The model under review builds one solid part; all positions refer to its coordinate system, in mm. Face numbers are marked on the shaded views. A direction names the side the tool comes from. Coordinates: 2 decimals unless noted, no trailing zeros. Loops run counter-clockwise (first coordinate to the right, second up) from the corner with the lowest first, then second, coordinate; pieces in that order, holes last. Notation, with made-up numbers: M 12.5,54.5 L 42.5,54.5 A37 cw 42.5,93.5 Z; hole C -36,85.5 d7. An arc over 180 degrees is marked long. Return JSON: item names as keys, results as strings.
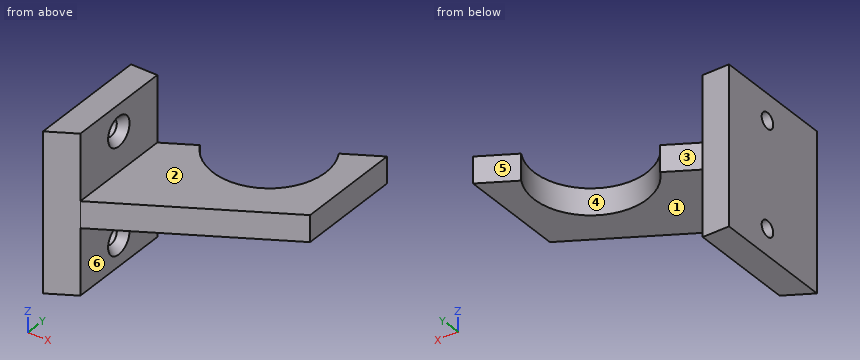
Autodesk Inventor part; units mm, degrees
ref_plane "YZ Plane" through (0, 0, 0) normal (1, 0, 0) x (0, 1, 0)
ref_plane "XZ Plane" through (0, 0, 0) normal (0, 1, 0) x (-1, 0, 0)
ref_plane "XY Plane" through (0, 0, 0) normal (0, 0, 1) x (1, 0, 0)
sketch "Sketch5" plane through (0, 0, 0) normal (0, 0, 1) x (1, 0, 0)
  line L0 (0, 0) -> (6.35, 0)
  line L1 (6.35, 0) -> (6.35, 25.4)
  line L2 (6.35, 25.4) -> (0, 25.4)
  line L3 (0, 25.4) -> (0, 0)
  dimension "d21" = 25.4
  dimension "d22" = 6.35
extrude "Extrusion3" add sketch "Sketch5" against normal mid plane 38.1
sketch "Sketch6" plane through (0, 0, 0) normal (0, 0, 1) x (1, 0, 0)
  line L0 (6.35, 25.4) -> (6.35, 0)
  line L1 (0, 25.4) -> (6.35, 25.4)
  line L2 (6.35, 0) -> (0, 0)
  line L3 (0, 0) -> (0, 25.4)
  line L4 (6.35, 0) -> (45.4025, 22.547)
  line L5 (6.35, 0) -> (51.4439, 0) construction
  line L6 (45.4025, 47.947) -> (45.4025, 22.547)
  arc A0 (13.5766, 29.5723) -> (37.2234, 43.2248) centre (25.4, 36.3985) ccw
  line L7 (6.35, 25.4) -> (13.5766, 29.5723)
  line L8 (37.2234, 43.2248) -> (45.4025, 47.947)
  dimension "d25" = 30
  dimension "d26" = 27.305
  dimension "d29" = 6.35
  dimension "d30" = 25.4
  dimension "d33" = 0
extrude "Extrusion4" add sketch "Sketch6" along normal mid plane 6.35 contours L7 A0 L8 L6 L4 L0
sketch "Sketch7" plane through (6.35, 0, 19.05) normal (1, 0, 0) x (0, 0, -1)
  line L0 (38.1, 25.4) -> (0, 25.4) construction
  line L1 (6.35, 25.4) -> (6.35, 0) construction
  line L2 (31.75, 25.4) -> (31.75, 0) construction
  line L3 (0, 0) -> (0, 25.4) construction
  line L4 (38.1, 25.4) -> (38.1, 0) construction
  line L5 (0, 0) -> (15.875, 0)
  line L6 (22.225, 0) -> (38.1, 0)
  point P0 (19.05, 0)
  point P1 (6.35, 12.7)
  point P2 (31.75, 12.7)
  dimension "d34" = 6.35
  dimension "d35" = 6.35
sketch "Sketch8" plane through (0, 0, 0) normal (0, 0, 1) x (1, 0, 0)
  line L0 (0, 0) -> (0, 25.4)
  line L1 (6.35, 0) -> (0, 0)
  line L2 (45.4025, 22.547) -> (6.35, 0)
  line L3 (0, 0) -> (6.35, 0)
  line L4 (0, -3.6662) -> (6.35, 0)
  line L5 (0, 0) -> (0, -3.6662)
extrude "Extrusion5" add sketch "Sketch8" along normal mid plane 38.1
hole "Hole3" at (6.35, 12.7, 12.7) at (6.35, 12.7, -12.7) direction (-1, 0, 0) diameter 3.81 end through all countersink diameter 7.0866 countersink angle 82
equation "\"d21\" = supportHeight"
equation "\"d22\" = supportWidth"
equation "\"d23\" = totalScrewHoldWidth"
equation "\"d25\" = supportAngle"
equation "\"d26\" = pipeDiameter"
equation "\"d30\" = distanceFromWallToPipeCenter"
equation "\"d31\" = supportWidth"
equation "\"d47\" = totalScrewHoldWidth"
equation "\"pipeDiameter\" = 27.305"
equation "\"distanceFromWallToPipeCenter\" = 25.4"
equation "\"supportHeight\" = 25.4"
equation "\"supportWidth\" = 6.35"
equation "\"screwHoldDepth\" = 6.35"
equation "\"totalScrewHoldWidth\" = 38.1"
equation "\"screwPositionFromTop\" = 6.35"
equation "\"supportAngle\" = 30deg"
properties part number "PipeSupport-1_00-030"
1. Add section C-C on y = 27. Give the boundary of the cut face in (x, z) (1 decimal), plus the area to 3 significant figures.
Check values:
{"outline": "M 9.1,-3.2 L 15.5,-3.2 L 15.5,3.2 L 9.1,3.2 Z; M 35.3,-3.2 L 45.4,-3.2 L 45.4,3.2 L 35.3,3.2 Z", "area": "105 mm²"}
2. Add section D-D on y = 20. Give the boundary of the cut face in (x, z) (3 decimals).
Check values:
{"outline": "M 0,-19.05 L 6.35,-19.05 L 6.35,-3.175 L 40.991,-3.175 L 40.991,3.175 L 6.35,3.175 L 6.35,19.05 L 0,19.05 Z"}
3. To check wall thickness, follow line 1 (Z direction, x = 1.9, y = 12.7) (3 decimals); line 2 (Z direction, x = 15, y = 18.5) (3 decimals); line 3 (Y direction, x = 2.7, z = -12.7) (3 decimals). State the ranges of each line that lie inside material, in increasing order.
Check values:
{"line 1": "-19.05 to -14.605, -10.795 to 10.795, 14.605 to 19.05", "line 2": "-3.175 to 3.175", "line 3": "-2.107 to 10.795, 14.605 to 25.4"}
4. The part is to be moulded in two halves that separate along X. For the marked faces 4, 5 and 6, say which applies: released by +X, released by -X, zero draft, split by the parting line, or undercut.
Check values:
{"face 4": "undercut", "face 5": "released by -X", "face 6": "released by +X"}
5. Add section A-A on z = 12.7. Give the boundary of the cut face in (x, y) (3 decimals).
Check values:
{"outline": "M 0,-3.666 L 6.35,0 L 6.35,9.157 L 4.465,10.795 L 0,10.795 Z; M 0,14.605 L 4.465,14.605 L 6.35,16.243 L 6.35,25.4 L 0,25.4 Z"}
6. Machinability: for the marked faces 1, 2 and 3, which of the approach directions +Z, -Z, +X, -X, +Y, -Y give a long, thin tool a straight path to every point of the face, cutting with its end or side? Answer none if there is none.
Check values:
{"face 1": "-Z, +X, +Y, -Y", "face 2": "+Z, +X, +Y, -Y", "face 3": "+Z, -Z, -X, +Y"}
7. Add section B-B on y = 12.7. Give the boundary of the cut face in (x, z) (3 decimals).
Check values:
{"outline": "M 0,-19.05 L 6.35,-19.05 L 6.35,-16.243 L 4.465,-14.605 L 0,-14.605 Z; M 0,-10.795 L 4.465,-10.795 L 6.35,-9.157 L 6.35,-3.175 L 28.347,-3.175 L 28.347,3.175 L 6.35,3.175 L 6.35,9.157 L 4.465,10.795 L 0,10.795 Z; M 0,14.605 L 4.465,14.605 L 6.35,16.243 L 6.35,19.05 L 0,19.05 Z"}
8. Insertion check: pin 1 Ø11.5 at (x, y) = (27.5, 22) entering from -Z (3 decimals); pin 2 Ø8 at (x, y) = (17, 20.5) entering from +Z (3 decimals); pin 3 Ø5 at (x, z) = (37, 4) entering from +Y; pin 4 Ø4 at (x, z) = (9, 7) entering from -Y. Each pin has a flat end and moves straight along its axis. Give the tip position at first contact, or say it passes through.
Check values:
{"pin 1": "z = -3.175", "pin 2": "z = 3.175", "pin 3": "y = 44.46", "pin 4": "through"}
